Source: CAD feature listing. Evaluate the final solid. Frame: model axes, mm. Face numbers are marked on the shaded views. A direction names the side the tool comes from. Coordinates: 2 decimals unless noted, no trailing zeros. Write each loop counter-clockwise with the first axis right and the second up, starting at its lowest first coordinate (ties: lowest second). Pieces come first, ordered by that corner, then holes. Notation, with made-up numbers: M 81.5,-7 L 112.5,-7 A13 ccw 112.5,8 Z; hole C -16.75,-39 d10. An arc over 180 degrees is marked long. Write item = value, one per line. Start each with the question number.
1. Section query A-A (z = 6). Output: boundary loops of the cut face in (x, y).
2. Pull-direction query (X, two-part tool) for the marked faces 1, 2 and 3; classes: pulls with the +X half, pulls with the -X half, needs draft (parallel to the pull), parting line crosses it, or undercut.
3. Pin query (flat end, axial travel): pin 1 Ø8 at (x, y) = (-37, -39) entering from -Z; pin 2 Ø5 at (x, y) = (0, -23.5) entering from +Z; pin 3 Ø12 at (x, y) = (-46.5, 12) entering from +Z. Return the tip coordinate at first contact, or that it passes through.
4. Access query for the marked faces 4 and 5. Directions: +Z, -Z, +X, -X, +Y, -Y. A direction counts if a zero-diameter tool reaches every point of the face in a straight line with its end or side. Return the directions, or none.
5. Section query C-C (x = -51.5). Output: boundary loops of the cut face in (y, z).
6. Section query D-D (y = -42). Output: boundary loops of the cut face in (x, z).
7. Section query B-B (y = 5.5). Output: boundary loops of the cut face in (x, z), then the cut area to 3 significant figures.
8. Line query: line 1 along X through (y, z) = (-19.5, 12.5); line 2 along Y through (x, z) = (-29, 6); line 3 along Y through (x, z) = (0, 13). Output: solid intervals per line, ascending.
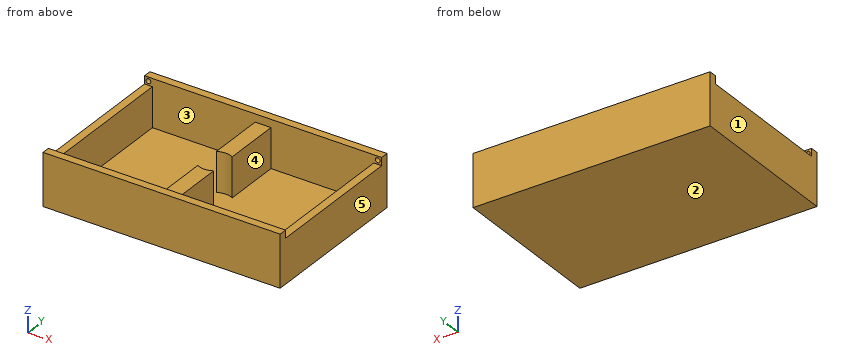
```python
from build123d import *

# Parameters (mm, degrees)
F0_W     = 150
F0_H     = 100
F1_DEPTH = 33
F2_W     = 65
F2_H     = 90
F3_DEPTH = 30
F4_W     = 5
F4_H     = 90
F5_DEPTH = 5
F7_R     = 10
F8_DEPTH = 25


with BuildPart() as f1:
    # F0 (on Top) → F1 (new body)
    with BuildSketch(Plane.XY):
        Rectangle(F0_W, F0_H)
    extrude(amount=F1_DEPTH)

    # F2 (on face) → F3 (cut)
    with BuildSketch(Plane.XY.offset(33)):
        with Locations((-37.5, 0)):
            Rectangle(F2_W, F2_H)
        with Locations((37.5, 0)):
            Rectangle(F2_W, F2_H)
    extrude(amount=-F3_DEPTH, mode=Mode.SUBTRACT)

    # F4 (on face) → F5 (cut)
    with BuildSketch(Plane.XY.offset(33)):
        with Locations((-72.5, 0)):
            Rectangle(F4_W, F4_H)
        with Locations((-2.5, 0)):
            Rectangle(F4_W, F4_H)
        with Locations((2.5, 0)):
            Rectangle(F4_W, F4_H)
        with Locations((72.5, 0)):
            Rectangle(F4_W, F4_H)
    extrude(amount=-F5_DEPTH, mode=Mode.SUBTRACT)

    # F7 (on face) → F8 (cut, through all)
    with BuildSketch(Plane.XY.offset(28)):
        Circle(F7_R)
    extrude(amount=-F8_DEPTH, mode=Mode.SUBTRACT)

    # F6 (on face) → F9 (revolve, cut)
    with BuildSketch(Plane.XZ.offset(-45)):
        with BuildLine():
            Line((-72.5, 29), (-72.5, 32))
            ThreePointArc((-72.5, 32), (-74, 30.5), (-72.5, 29))
        make_face()
    revolve(axis=Axis((-72.5, 45, 30.5), (0, 0, -1)), mode=Mode.SUBTRACT)

    # F10: F1 across plane


with BuildPart() as f1_1:
    add(f1.part)
    add(f1.part.mirror(Plane.YZ), mode=Mode.INTERSECT)

    # F11: F1 across plane


with BuildPart() as f1_2:
    add(f1_1.part)
    add(f1_1.part.mirror(Plane.XZ), mode=Mode.INTERSECT)


solid = f1_2.part
```
Results are:
q1.outline = M -75,-50 L 75,-50 L 75,50 L -75,50 Z; hole M -70,-45 L -5,-45 L -5,-8.66 A10 ccw 5,-8.66 L 5,-45 L 70,-45 L 70,45 L 5,45 L 5,8.66 A10 ccw -5,8.66 L -5,45 L -70,45 Z
q2.face_1 = pulls with the -X half
q2.face_2 = needs draft
q2.face_3 = undercut
q3.pin_1 = 0
q3.pin_2 = 28
q3.pin_3 = 3
q4.face_4 = +Z
q4.face_5 = +Z, -Z, +X, +Y, -Y
q5.outline = M -50,0 L 50,0 L 50,33 L 45,33 L 45,3 L -45,3 L -45,33 L -50,33 Z
q6.outline = M -75,0 L 75,0 L 75,28 L 70,28 L 70,3 L 5,3 L 5,28 L -5,28 L -5,3 L -70,3 L -70,28 L -75,28 Z
q7.outline = M -75,0 L 75,0 L 75,28 L 70,28 L 70,3 L -70,3 L -70,28 L -75,28 Z
q7.area = 700 mm^2
q8.line_1 = -75 to -70, -5 to 5, 70 to 75
q8.line_2 = -50 to -45, 45 to 50
q8.line_3 = -50 to -10, 10 to 50
